The listing builds one solid part. Answer for the finished solid, in the listing's coordinates (mm). A direction names the side the tool comes from. Give positions to 0.01 mm unless a question says otherwise; leave off trailing zeros. Order: outer loops, then holes, each group sorted by start corner. A loop starts at its lowest first (then second) coordinate and runs counter-clockwise, first axis right, second up.
```python
from build123d import *

# Parameters (mm, degrees)
SKETCH1_W           = 69.85
SKETCH1_H           = 44.45
SKETCH1_R           = 3.2639
SKETCH1_R_2         = 3.5
BOSS_EXTRUDE1_DEPTH = 3.175
SKETCH2_R           = 4.5
CUT_EXTRUDE1_DEPTH  = 2


with BuildPart() as part:
    # Sketch1 → Boss-Extrude1 (new body)
    with BuildSketch(Plane(origin=(0, 0, 0), x_dir=(1, 0, 0), z_dir=(0, 1, 0))):
        with Locations((34.925, 22.225)):
            Rectangle(SKETCH1_W, SKETCH1_H)
        with Locations((9.525, 34.925)):
            Circle(SKETCH1_R, mode=Mode.SUBTRACT)
        with Locations((60.325, 34.925)):
            Circle(SKETCH1_R, mode=Mode.SUBTRACT)
        with Locations((9.525, 9.525)):
            Circle(SKETCH1_R, mode=Mode.SUBTRACT)
        with Locations((60.325, 9.525)):
            Circle(SKETCH1_R, mode=Mode.SUBTRACT)
        with Locations((44.925, 32.225)):
            Circle(SKETCH1_R_2, mode=Mode.SUBTRACT)
        with Locations((34.925, 32.225)):
            Circle(SKETCH1_R_2, mode=Mode.SUBTRACT)
        with Locations((24.925, 32.225)):
            Circle(SKETCH1_R_2, mode=Mode.SUBTRACT)
        with Locations((34.925, 22.225)):
            Circle(SKETCH1_R_2, mode=Mode.SUBTRACT)
        with Locations((24.925, 22.225)):
            Circle(SKETCH1_R_2, mode=Mode.SUBTRACT)
        with Locations((34.925, 12.225)):
            Circle(SKETCH1_R_2, mode=Mode.SUBTRACT)
        with Locations((24.925, 12.225)):
            Circle(SKETCH1_R_2, mode=Mode.SUBTRACT)
        with Locations((44.925, 22.225)):
            Circle(SKETCH1_R_2, mode=Mode.SUBTRACT)
        with Locations((44.925, 12.225)):
            Circle(SKETCH1_R_2, mode=Mode.SUBTRACT)
    extrude(amount=BOSS_EXTRUDE1_DEPTH)

    # Sketch2 → Cut-Extrude1 (cut)
    with BuildSketch(Plane(origin=(0, 3.175, 0), x_dir=(1, 0, 0), z_dir=(0, 1, 0))):
        with Locations((44.925, 12.225)):
            Circle(SKETCH2_R)
        with Locations((34.925, 12.225)):
            Circle(SKETCH2_R)
        with Locations((24.925, 12.225)):
            Circle(SKETCH2_R)
        with Locations((34.925, 22.225)):
            Circle(SKETCH2_R)
        with Locations((24.925, 22.225)):
            Circle(SKETCH2_R)
        with Locations((34.925, 32.225)):
            Circle(SKETCH2_R)
        with Locations((24.925, 32.225)):
            Circle(SKETCH2_R)
        with Locations((44.925, 22.225)):
            Circle(SKETCH2_R)
        with Locations((44.925, 32.225)):
            Circle(SKETCH2_R)
    extrude(amount=-CUT_EXTRUDE1_DEPTH, mode=Mode.SUBTRACT)


solid = part.part
```
1) For a pull along Z with two mould halves and no side action, classify faces 1 (the flat face through (38, 1.175, -20)), 2 (the flat face through (34, 2, -44.45)), 3 (the flat face through (0, 2, -22)) as +Z half, -Z half, draft (parallel to the pull), parting line (faces both ways), or undercut.
Geometry says:
face 1: undercut
face 2: -Z half
face 3: draft
2) Find section B-B (x = 9.5). Write down the section's boundary in (y, z) (3 decimals), then the cut area to 3 significant figures.
Geometry says:
outline: (0, -44.45) - (3.175, -44.45) - (3.175, -38.189) - (0, -38.189) - close; (0, -31.661) - (3.175, -31.661) - (3.175, -12.789) - (0, -12.789) - close; (0, -6.261) - (3.175, -6.261) - (3.175, 0) - (0, 0) - close
area: 99.7 mm2
3) Find section D-D (y = 2.3). Count the separate pieces of the cut face and the enclosed holes in it, then the cut area to 3 significant figures.
Geometry says:
separate pieces: 1
enclosed holes: 13
area: 2,400 mm2
4) Find section C-C (z = -19.5). Write down the section's boundary in (x, y) (3 decimals).
Geometry says:
outline: (0, 0) - (22.729, 0) - (22.729, 1.175) - (21.344, 1.175) - (21.344, 3.175) - (0, 3.175) - close; (27.121, 0) - (32.729, 0) - (32.729, 1.175) - (31.344, 1.175) - (31.344, 3.175) - (28.506, 3.175) - (28.506, 1.175) - (27.121, 1.175) - close; (37.121, 0) - (42.729, 0) - (42.729, 1.175) - (41.344, 1.175) - (41.344, 3.175) - (38.506, 3.175) - (38.506, 1.175) - (37.121, 1.175) - close; (47.121, 0) - (69.85, 0) - (69.85, 3.175) - (48.506, 3.175) - (48.506, 1.175) - (47.121, 1.175) - close
5) A tool of negligible diameter and unlimited length cuts with its end or side. For faces 4 (the cylindrical face through (63.34, 1.57, -33.67)), 5 (the cylindrical face through (49.217, 2.189, -13.577)), from which of +Z, -Z, +X, -X, +Y, -Y can it reach the whole face along a straight path? Write none if from no direction.
Geometry says:
face 4: +Y, -Y
face 5: +Y
6) Find section A-A (x = 34). Write down the section's boundary in (y, z) (3 decimals), then the cut area to 3 significant figures.
Geometry says:
outline: (0, -44.45) - (3.175, -44.45) - (3.175, -36.629) - (1.175, -36.629) - (1.175, -35.601) - (0, -35.601) - close; (0, -28.849) - (1.175, -28.849) - (1.175, -27.821) - (3.175, -27.821) - (3.175, -26.629) - (1.175, -26.629) - (1.175, -25.601) - (0, -25.601) - close; (0, -18.849) - (1.175, -18.849) - (1.175, -17.821) - (3.175, -17.821) - (3.175, -16.629) - (1.175, -16.629) - (1.175, -15.601) - (0, -15.601) - close; (0, -8.849) - (1.175, -8.849) - (1.175, -7.821) - (3.175, -7.821) - (3.175, 0) - (0, 0) - close
area: 64.5 mm2
7) Straight lines are drawn through the part: probe 1 along Z at (x, y) = (60.5, 2.5); probe 2 along X at (y, z) = (1.1, -14); probe 3 along Z at (x, y) = (32, 0.6). For each, find the intervals that lie inside material, in ascending order.
Geometry says:
probe 1: z = -44.45 to -38.18, -31.67 to -12.78, -6.27 to 0
probe 2: x = 0 to 21.91, 27.94 to 31.91, 37.94 to 41.91, 47.94 to 69.85
probe 3: z = -44.45 to -34.15, -30.3 to -24.15, -20.3 to -14.15, -10.3 to 0
8) Given P1, Ø6.5, axis at x = 44.925, z = -32.225, coming from the -Y side, flat-ended and moving along its own axis, determine where the tip first touches the part or whether it passes through.
Geometry says:
P1: passes through
